Source: three-view drawing plus pictorial views. Frame: mm from the lowest corner of the part. A direction names the side the tool comes from. Give positions to 0.01 mm unless a question says otherwise; leave off trailing zeros. Write each loop counter-clockwise with the first axis right and the second up, starting at its lowest first coordinate (ties: lowest second). Pieces come first, ordered by that corner, then holes. Notation, with made-up numbers: (23, 31.25) -> (62, 31.25) arc R30 cw to (62, 55.25) -> close; hole circle Ø8 at (34, 29). An arc over 180 degrees is marked (long way). Answer in a Markdown table with one row per item. Add a question column.
Item 1: Material intervals for probe 1 along X at (y, z) = (15, 18.5); probe 2 along Z at (x, y) = (3.75, 13); probe 3 along X at (y, z) = (8.15, 12.5), sorted ascending. Write a range as from..to.
Item 2: First-contact query: P1, Ø5, axis at y = 12.5, z = 21.5, coming from the +X side; P2, Ø1, axis at x = 2, z = 6.5, coming from the +Y side (3 decimals); P3, Ø4, axis at x = 6.5, z = 11.5, coming from the +Y side; P4, Ø12, axis at y = 17.5, z = 10, coming from the +X side. Flat tips, straight axial feed; report the tip coordinate or a pass-through.
Item 3: Access query for the marked faces 1 and 2. Directions: +Z, -Z, +X, -X, +Y, -Y. A direction counts if a zero-diameter tool reaches every point of the face in a straight line with its end or side. Return the directions, or none.
Item 4: Section query D-D on y = 16.5. Output: boundary loops of the cut face in (x, z).
Item 5: Section query A-A on y = 12.5. Output: boundary loops of the cut face in (x, z), plus the area to 3 significant figures.
Item 6: Draft query along Y for the marked faces 3, 4 and 5. Return one class per face: +Y half, -Y half, draft (parallel to the pull), parting line (faces both ways), or undercut.
Item 7: Section query C-C on x = 2. Output: boundary loops of the cut face in (y, z), plus the area to 3 significant figures.
Item 8: Section query B-B on z = 12.75. Output: boundary loops of the cut face in (x, y), plus the area to 3 significant figures.
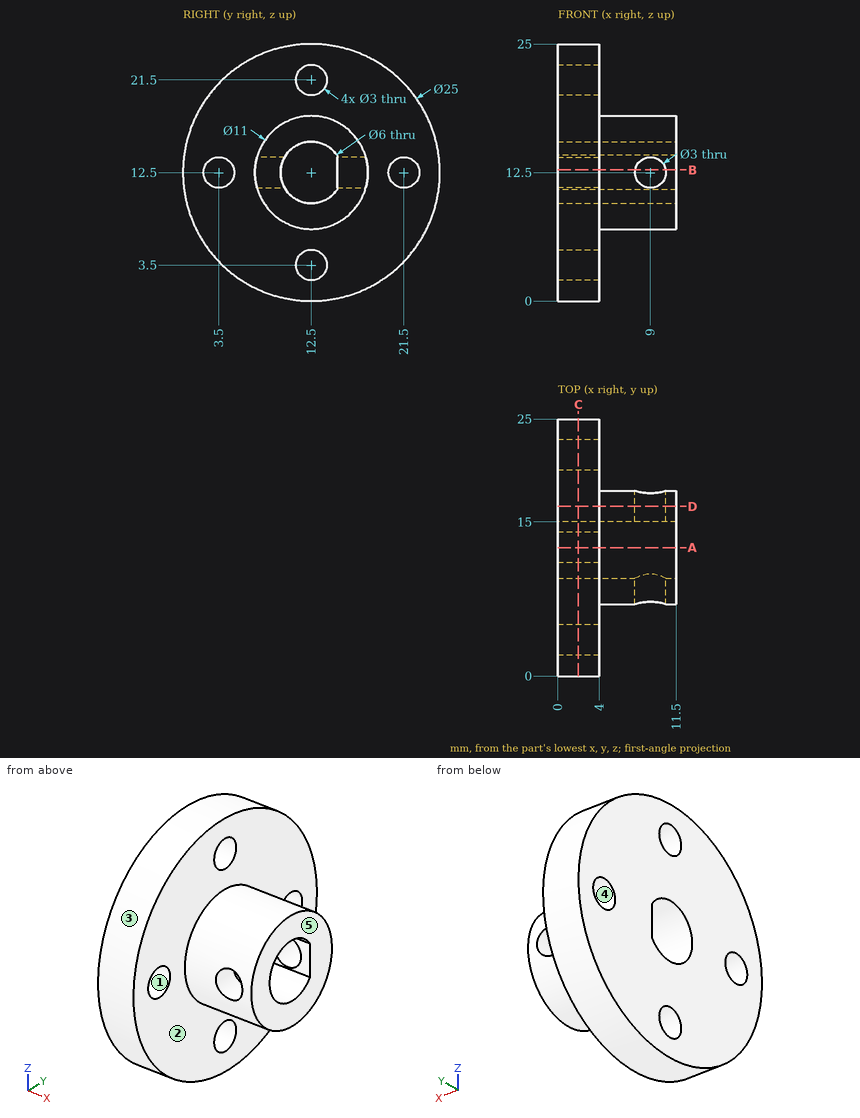
Findings below:
| question | item | result |
|---|---|---|
| 1 | probe 1 | x = 0..4 |
| 1 | probe 2 | z = 0.01..2.09, 4.91..9.54, 15.46..20.09, 22.91..24.99 |
| 1 | probe 3 | x = 0..7.5, 10.5..11.5 |
| 2 | P1 | stops at x = 4 |
| 2 | P2 | stops at y = 23.725 |
| 2 | P3 | stops at y = 18 |
| 2 | P4 | stops at x = 11.5 |
| 3 | face 1 | +X, -X |
| 3 | face 2 | +X |
| 4 | outline | (0, 0.66) -> (4, 0.66) -> (4, 8.73) -> (11.5, 8.73) -> (11.5, 16.27) -> (4, 16.27) -> (4, 24.34) -> (0, 24.34) -> close; hole circle Ø3 at (9, 12.5) |
| 5 | outline | (0, 0) -> (4, 0) -> (4, 2) -> (0, 2) -> close; (0, 5) -> (4, 5) -> (4, 7) -> (11.5, 7) -> (11.5, 9.5) -> (0, 9.5) -> close; (0, 15.5) -> (11.5, 15.5) -> (11.5, 18) -> (4, 18) -> (4, 20) -> (0, 20) -> close; (0, 23) -> (4, 23) -> (4, 25) -> (0, 25) -> close |
| 5 | area | 89.5 mm^2 |
| 6 | face 3 | parting line |
| 6 | face 4 | undercut |
| 6 | face 5 | draft |
| 7 | outline | circle Ø25 at (12.5, 12.5); hole circle Ø3 at (3.5, 12.5); hole circle Ø3 at (12.5, 3.5); hole circle Ø3 at (12.5, 21.5); hole (15, 10.84) -> (15, 14.16) arc R3 ccw (long way) to start; hole circle Ø3 at (21.5, 12.5) |
| 7 | area | 435 mm^2 |
| 8 | outline | (0, 0) -> (4, 0) -> (4, 2.02) -> (0, 2.02) -> close; (0, 4.98) -> (4, 4.98) -> (4, 7.01) -> (7.52, 7.01) -> (7.52, 9.51) -> (0, 9.51) -> close; (0, 15) -> (7.52, 15) -> (7.52, 17.99) -> (4, 17.99) -> (4, 20.02) -> (0, 20.02) -> close; (0, 22.98) -> (4, 22.98) -> (4, 25) -> (0, 25) -> close; (10.48, 7.01) -> (11.5, 7.01) -> (11.5, 9.51) -> (10.48, 9.51) -> close; (10.48, 15) -> (11.5, 15) -> (11.5, 17.99) -> (10.48, 17.99) -> close |
| 8 | area | 79.3 mm^2 |
